The figure shows three views and two pictorial views of one solid part (mm, origin at its lowest corner). Answer the questions. Round coordinates to 2 decimals unless told otherwise and drop trailing zeros. Order: outer loops, then holes, each group sorted by start corner. A loop starts at its lowest first (then second) coordinate and runs counter-clockwise, first axis right, second up. Notation, with made-up numbers: (-7.5, 56.25) - (13.5, 56.25) arc R17 ccw to (13.5, 60.25) - close; hole circle Ø4 at (60, 42). An arc over 180 degrees is marked (long way). Answer in a Markdown table with one row per item.
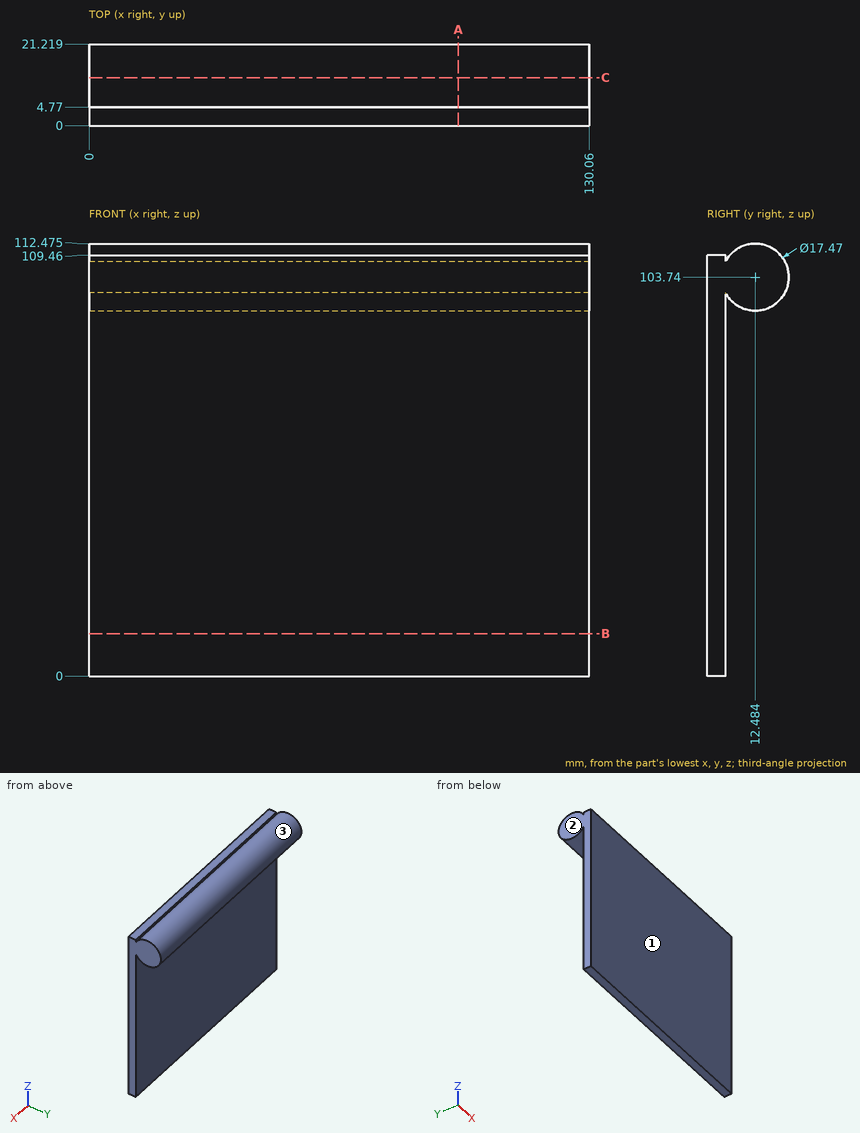
1) The mould has two halves that part along Y. Classify the marked faces 1, 2 and 3: released by +Y, released by -Y, zero draft, split by the parting line, or undercut.
Filled in:
| item | result |
|---|---|
| face 1 | released by -Y |
| face 2 | zero draft |
| face 3 | undercut |
2) Find section B-B, the plane z = 11. Give the vertices of the cut face in (x, y).
Filled in:
| item | result |
|---|---|
| outline | (0, 0) - (130.06, 0) - (130.06, 4.77) - (0, 4.77) - close |
3) Find section C-C, the plane y = 12.5. Give the vertices of the cut face in (x, z) (1 decimal).
Filled in:
| item | result |
|---|---|
| outline | (0, 95) - (130.1, 95) - (130.1, 112.5) - (0, 112.5) - close |
4) Find the intervals of material crossed by probe 1 along Y at (x, z) = (60, 47.5); probe 2 along Z at (x, y) = (43.5, 2.75); probe 3 along Z at (x, y) = (17, 19) (1 decimal), in increasing order. Write a range as from..to.
Filled in:
| item | result |
|---|---|
| probe 1 | y = 0..4.77 |
| probe 2 | z = 0..109.46 |
| probe 3 | z = 97.9..109.6 |
5) Each of these flat-tipped pins is pushed along its axis until it touches: pin 1 (4 mm diameter, centred on x = 78, y = 3, fed in from +Z); pin 2 (2 mm diameter, centred on x = 31, z = 86.5, fed in from +Y); pin 3 (1.5 mm diameter, centred on x = 63.5, y = 19, fed in from +Z). Where does it stop, or does it pass through?
Filled in:
| item | result |
|---|---|
| pin 1 | stops at z = 109.46 |
| pin 2 | stops at y = 4.77 |
| pin 3 | stops at z = 110.3 |
6) Find section A-A, the plane x = 96. Give the vertices of the cut face in (y, z) (1 decimal), then the cut area to 3 significant figures.
Filled in:
| item | result |
|---|---|
| outline | (0, 0) - (4.8, 0) - (4.8, 99.6) arc R8.7 ccw (long way) to (4.8, 107.8) - (4.8, 109.5) - (0, 109.5) - close |
| area | 756 mm^2 |
